Input: dimensioned drawing with shaded views. Units: mm. Origin: part minimum x, y, z. Coordinates: 2 decimals unless noted, no trailing zeros. Order: outer loops, then holes, each group sorted by start corner. A loop starts at its lowest first (then second) coordinate and runs counter-clockwise, first axis right, second up.
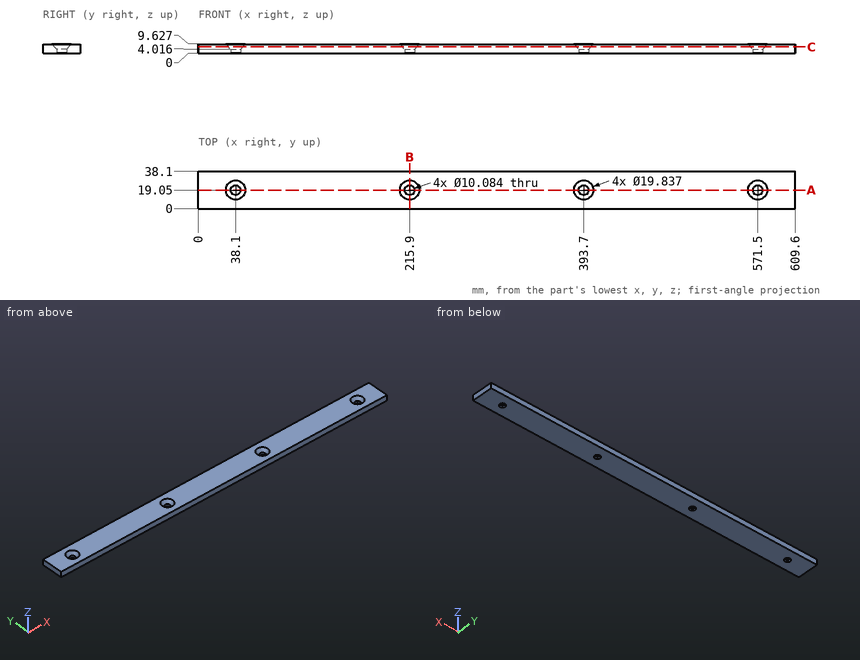
1. Section query B-B on x = 215.9. Return loops of the section in (y, z), plus the area to 3 significant figures.
Findings:
outline: (0, 0) - (14.01, 0) - (14.01, 4.02) - (9.13, 9.63) - (0, 9.63) - close; (24.09, 0) - (38.1, 0) - (38.1, 9.63) - (28.97, 9.63) - (24.09, 4.02) - close
area: 242 mm2
2. Section query A-A on y = 19.05. Return loops of the section in (x, z), plus the area to 3 significant figures.
Findings:
outline: (0, 0) - (33.06, 0) - (33.06, 4.02) - (28.18, 9.63) - (0, 9.63) - close; (43.14, 0) - (210.86, 0) - (210.86, 4.02) - (205.98, 9.63) - (48.02, 9.63) - (43.14, 4.02) - close; (220.94, 0) - (388.66, 0) - (388.66, 4.02) - (383.78, 9.63) - (225.82, 9.63) - (220.94, 4.02) - close; (398.74, 0) - (566.46, 0) - (566.46, 4.02) - (561.58, 9.63) - (403.62, 9.63) - (398.74, 4.02) - close; (576.54, 0) - (609.6, 0) - (609.6, 9.63) - (581.42, 9.63) - (576.54, 4.02) - close
area: 5,370 mm2
3. Pin query (flat end, axial travel): P1, Ø13, axis at x = 215.9, y = 19.05, coming from the -Z side; P2, Ø11.5, axis at x = 393.7, y = 19.05, coming from the +Z side; P3, Ø8, axis at x = 38.1, y = 19.05, coming from the +Z side. Return the tip coordinate at first contact, or that it passes through.
Findings:
P1: stops at z = 0
P2: stops at z = 4.83
P3: passes through
4. Section query C-C on z = 6.75. Return loops of the section in (x, y).
Findings:
outline: (0, 0) - (609.6, 0) - (609.6, 38.1) - (0, 38.1) - close; hole circle Ø14.84 at (38.1, 19.05); hole circle Ø14.84 at (215.9, 19.05); hole circle Ø14.84 at (393.7, 19.05); hole circle Ø14.84 at (571.5, 19.05)
5. Ray query, line 1 (X direction, y = 19.05, z = 1.1); line 2 (Y direction, x = 38.1, z = 2.6); line 3 (X direction, y = 18, z = 3.25). Return the intervals inside material, ascending.
Findings:
line 1: x = 0 to 33.06, 43.14 to 210.86, 220.94 to 388.66, 398.74 to 566.46, 576.54 to 609.6
line 2: y = 0 to 14.01, 24.09 to 38.1
line 3: x = 0 to 33.17, 43.03 to 210.97, 220.83 to 388.77, 398.63 to 566.57, 576.43 to 609.6
